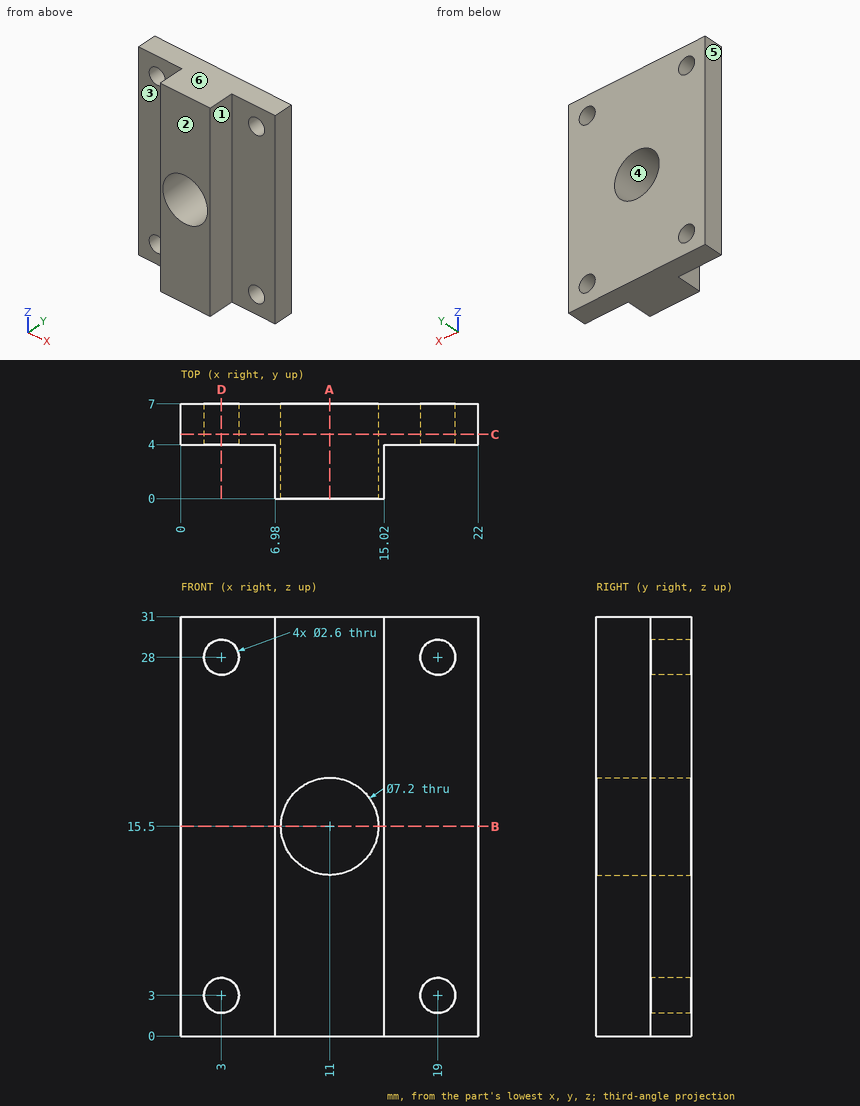
Geometry check sheet. Reference: drawing and pictorial views, mm from the part's lowest x, y, z. A direction names the side the tool comes from. Round coordinates to 2 decimals unless told otherwise and drop trailing zeros. Write each loop counter-clockwise with the first axis right and the second up, starting at its lowest first coordinate (ties: lowest second). Pieces come first, ordered by that corner, then holes.
(1) Section check B-B (z = 15.5). Enter the section's corners in (x, y).
Returned:
outline: (0, 4) - (6.98, 4) - (6.98, 0) - (7.4, 0) - (7.4, 7) - (0, 7) - close; (14.6, 0) - (15.02, 0) - (15.02, 4) - (22, 4) - (22, 7) - (14.6, 7) - close
(2) Section check C-C (y = 4.75). Enter the section's corners in (x, z).
Returned:
outline: (0, 0) - (22, 0) - (22, 31) - (0, 31) - close; hole circle Ø2.6 at (3, 3); hole circle Ø2.6 at (3, 28); hole circle Ø7.2 at (11, 15.5); hole circle Ø2.6 at (19, 3); hole circle Ø2.6 at (19, 28)
(3) Access from +Z, -Z, +X, -X, +Y, -Y to the whole of each face (thin tool, end or side, straight path). Record for the marked faces 1, 2 and 3.
Returned:
face 1: +Z, -Z, +X, -Y
face 2: +Z, -Z, +X, -X, -Y
face 3: +Z, -Z, -X, -Y
(4) Material ranges on line 1 (X direction, y = 5.1, z = 3); line 2 (Z direction, x = 19, y = 4.7); line 3 (Z direction, x = 11, y = 2.75), recorded low to high.
Returned:
line 1: x = 0 to 1.7, 4.3 to 17.7, 20.3 to 22
line 2: z = 0 to 1.7, 4.3 to 26.7, 29.3 to 31
line 3: z = 0 to 11.9, 19.1 to 31
(5) Section check D-D (x = 3). Enter the section's corners in (y, z), plus the area to 3 significant figures.
Returned:
outline: (4, 0) - (7, 0) - (7, 1.7) - (4, 1.7) - close; (4, 4.3) - (7, 4.3) - (7, 26.7) - (4, 26.7) - close; (4, 29.3) - (7, 29.3) - (7, 31) - (4, 31) - close
area: 77.4 mm2
(6) Section check A-A (x = 11). Enter the section's corners in (y, z), plus the area to 3 significant figures.
Returned:
outline: (0, 0) - (7, 0) - (7, 11.9) - (0, 11.9) - close; (0, 19.1) - (7, 19.1) - (7, 31) - (0, 31) - close
area: 167 mm2
(7) Depth check by flat-ended pin: pin 1 Ø2 at (x, z) = (3, 3) entering from +Y (3 decimals); pin 2 Ø7.5 at (x, z) = (20, 22) entering from -Y; pin 3 Ø3 at (y, z) = (1.5, 23.5) entering from -X; pin 4 Ø2 at (y, z) = (1.5, 14.5) entering from +X. Enter the tip coordinate at first touch or a pass-through.
Returned:
pin 1: passes through
pin 2: stops at y = 4
pin 3: stops at x = 6.98
pin 4: stops at x = 15.02
(8) Mould release check, pull along Z, two halves, no side actions. Record for the marked faces 4, 5 and 6: pulls with the +Z half, pulls with the -Z half, needs draft (parallel to the pull), parting line crosses it, or undercut.
Returned:
face 4: undercut
face 5: needs draft
face 6: pulls with the +Z half
